Input: dimensioned drawing with shaded views. Units: mm. Origin: part minimum x, y, z. A direction names the side the tool comes from. Coordinates: 2 decimals unless noted, no trailing zeros. Loops run counter-clockwise (first coordinate to the right, second up) from the corner with the lowest first, then second, coordinate; pieces in that order, holes last. Notation, with made-up numbers: (6.25, 25.25) - (21.25, 25.25) arc R19 cw to (21.25, 44.25) - close; hole circle Ø7 at (86.5, -9.5). An arc over 180 degrees is marked (long way). Use one line per item in the form item = value. Start each with the question number.
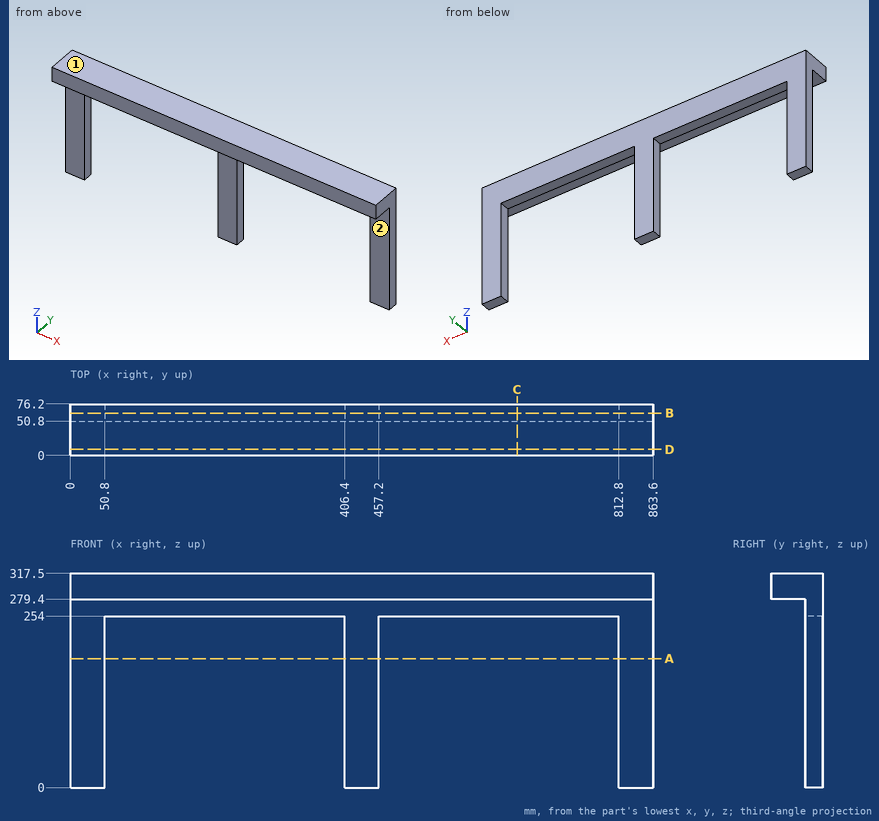
(1) Cut plane A-A, the plane z = 191. Output: boundary loops of the cut face in (x, y).
(2) Access query for the marked faces 1 and 2. Directions: +Z, -Z, +X, -X, +Y, -Y. A direction counts if a zero-diameter tool reaches every point of the face in a straight line with its end or side. Return the directions, or none.
(3) Contact query for flat-ended pins moving along their axis: pin 1 (12.5 mm diameter, centred on x = 716, y = 61, fed in from -Z); pin 2 (12 mm diameter, centred on y = 39.5, z = 173.5, fed in from +X); pin 3 (4 mm diameter, centred on x = 472.5, y = 19, fed in from -Z). Output: stop coordinate, or through.
(4) Cut plane C-C, the plane x = 662. Output: boundary loops of the cut face in (y, z).
(5) Material intervals for line 1 (X direction, y = 60.5, z = 213); line 2 (Y direction, x = 552.5, z = 266); line 3 (Z direction, x = 199, y = 39), sorted ascending.
(6) Cut plane B-B, the plane y = 62.5. Output: boundary loops of the cut face in (x, z), plus the area to 3 significant figures.
(7) Cut plane D-D, the plane y = 9. Output: boundary loops of the cut face in (x, z).
Recorded:
q1.outline = (0, 50.8) - (50.8, 50.8) - (50.8, 76.2) - (0, 76.2) - close; (406.4, 50.8) - (457.2, 50.8) - (457.2, 76.2) - (406.4, 76.2) - close; (812.8, 50.8) - (863.6, 50.8) - (863.6, 76.2) - (812.8, 76.2) - close
q2.face_1 = +Z, +X, -X, +Y, -Y
q2.face_2 = -Z, +X, -X, -Y
q3.pin_1 = 254
q3.pin_2 = through
q3.pin_3 = 279.4
q4.outline = (0, 279.4) - (50.8, 279.4) - (50.8, 254) - (76.2, 254) - (76.2, 317.5) - (0, 317.5) - close
q5.line_1 = 0 to 50.8, 406.4 to 457.2, 812.8 to 863.6
q5.line_2 = 50.8 to 76.2
q5.line_3 = 279.4 to 317.5
q6.outline = (0, 0) - (50.8, 0) - (50.8, 254) - (406.4, 254) - (406.4, 0) - (457.2, 0) - (457.2, 254) - (812.8, 254) - (812.8, 0) - (863.6, 0) - (863.6, 317.5) - (0, 317.5) - close
q6.area = 93,500 mm²
q7.outline = (0, 279.4) - (863.6, 279.4) - (863.6, 317.5) - (0, 317.5) - close
